Answer from the drawing. Dimensions are ordinates in mm from the lowest x, y and z of the part. A direction names the side the tool comes from. Give positions to 0.01 mm unless a question says otherwise; leave off trailing zeros. Order: outer loops, then holes, each group sorted by start corner. A loop starts at its lowest first (then second) coordinate and runs counter-clockwise, first axis right, second up.
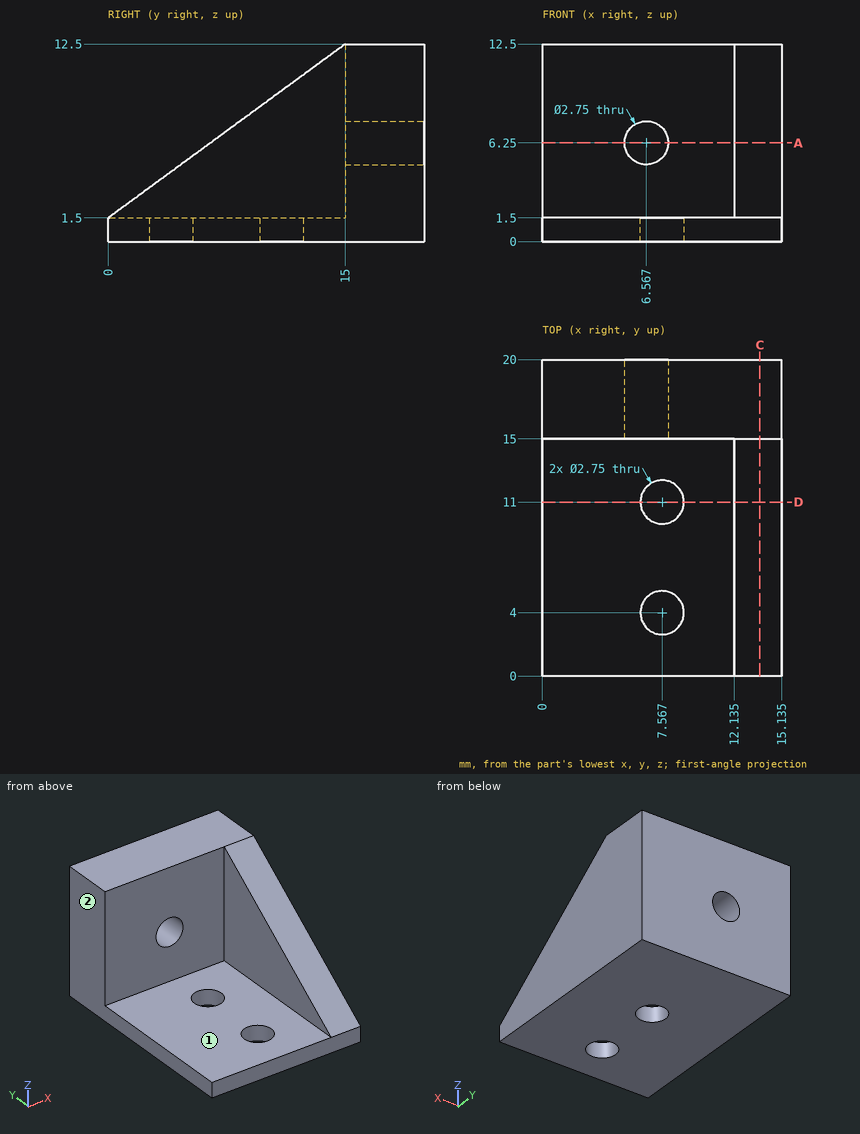
1) The part is cut by section A-A on z = 6.25. Determine the outline of the cut face in (x, y) (1 decimal).
Final values:
outline: (0, 15) - (5.2, 15) - (5.2, 20) - (0, 20) - close; (7.9, 15) - (12.1, 15) - (12.1, 6.5) - (15.1, 6.5) - (15.1, 20) - (7.9, 20) - close
2) Consider L1, parallel to X at y = 17.2, z = 6.25 (1 decimal); L2, parallel to Z at x = 10.5, y = 4.25; L3, parallel to Y at x = 4.75, z = 3.75. Determine where each line is inside the solid, lowest interval first.
Final values:
L1: x = 0 to 5.2, 7.9 to 15.1
L2: z = 0 to 1.5
L3: y = 15 to 20
3) The part is cut by section D-D on y = 11. Determine the outline of the cut face in (x, z) (1 decimal).
Final values:
outline: (0, 0) - (6.2, 0) - (6.2, 1.5) - (0, 1.5) - close; (8.9, 0) - (15.1, 0) - (15.1, 9.6) - (12.1, 9.6) - (12.1, 1.5) - (8.9, 1.5) - close
4) The part is cut by section C-C on x = 13.75. Determine the outline of the cut face in (y, z).
Final values:
outline: (0, 0) - (20, 0) - (20, 12.5) - (15, 12.5) - (0, 1.5) - close
5) A tool of negligible diameter and unlimited length cuts with its end or side. For the marked faces 1 and 2, from which of +Z, -Z, +X, -X, +Y, -Y can it reach the whole face along a straight path? Write none if from no direction.
Final values:
face 1: +Z, -X, -Y
face 2: +Z, -Z, -X, +Y, -Y
6) Given pin 1 (3 mm diameter, centred on y = 4.5, z = 3.5, fed in from -X) (1 decimal); pin 2 (2.5 mm diameter, centred on x = 7.57, y = 4, fed in from +Z); pin 3 (3.5 mm diameter, centred on x = 9, y = 8, fed in from +Z); pin 4 (1 mm diameter, centred on x = 12, z = 2.5, fed in from -Y) (1 decimal), each flat-ended and moving along its own axis, determine where each tip first touches the part or whether it passes through.
Final values:
pin 1: stops at x = 12.1
pin 2: passes through
pin 3: stops at z = 1.5
pin 4: stops at y = 0.7
